Input: part model. Units: mm. Frame: model coordinates. A direction names the side the tool comes from. Coordinates: 2 decimals unless noted, no trailing zeros. Loops run counter-clockwise (first coordinate to the right, second up) from the corner with the lowest first, then second, coordinate; pieces in that order, holes last.
Item 1: Reachability of faces 5 (the flat face through (-9.55, 41, 12)), 6 (the cylindrical face through (-17.435, 32.128, 3.838)), 7 (the flat face through (-6, 26, 10)), 8 (the flat face through (-3.032, 41, 7)) from +Z, -Z, +X, -X, +Y, -Y: full face, straight path, thin tool, end or side. Return the list, or none.
Item 2: Section D-D on z = 1.25. Return loops of the section in (x, y), and give its area (3 significant figures).
Item 3: Section B-B on y = 41. Return loops of the section in (x, z).
Item 4: Section A-A on z = 9.85. Return loops of the section in (x, y), and give its area (3 significant figures).
Item 5: Pull-direction query (Z, two-part tool) for faces 1 (the cylindrical face through (-6.337, 41.26, 11.833)), 2 (the flat face through (0.45, -4, 2)), 3 (the flat face through (-6, 41, 15)), 4 (the flat face through (-20, 16, 0)); classes: released by +Z, released by -Z, zero draft, split by the parting line, or undercut.
Item 6: Section C-C on x = -22.5. Return loops of the section in (y, z), and give its area (3 significant figures).
Item 7: Ray query, line 1 along Y through (x, z) = (-4, 6.75); line 2 along Y through (x, z) = (-3.5, 14.5); line 3 along Z through (x, y) = (-16, -2.5). Return the intervals inside material, ascending.
Item 8: Contact query for flat-ended pins moving along their axis: P1, Ø1.3, axis at y = 29, z = 10.5, coming from the +X side; P2, Ø7, axis at x = -5, z = 9, coming from the -Y side; P3, Ø18, axis at x = -22.05, y = 41, coming from the +Z side. Output: stop coordinate, or through.
```python
from build123d import *

# Parameters (mm, degrees)
F0_R       = 3.5
F0_R_2     = 10
F0_R_3     = 2
F1_DEPTH   = 4.7
F2_SIZE2   = 1.6781992624
F2_SIZE    = 2
F2_2_SIZE2 = 1.6781992624
F2_2_SIZE  = 2
F2_3_SIZE2 = 1.6781992624
F2_3_SIZE  = 2
F3_DEPTH   = 15
F0_R_4     = 4.75
F4_DEPTH   = 3
F5_R       = 2
F6_DEPTH   = 8


# Not quite as in the source:
# - a feature names something its author has since deleted; it is built from what else it names


with BuildPart() as f1:
    # F0 (on Top) → F1 (new body)
    with BuildSketch(Plane.XY):
        Polygon((-39.2612926662, 18.4351751247), (-14.0709569678, -26), (0.450202167, -26), (0.450202167, 18.6235290021), (-3.0323355459, 26), (-9.549797833, 26), (-9.549797833, 56), (-39.2612926662, 56), align=None)
        with Locations((-7.549797833, -21)):
            Circle(F0_R, mode=Mode.SUBTRACT)
        with Locations((-28.549797833, 21)):
            Circle(F0_R, mode=Mode.SUBTRACT)
        with Locations((-22.049797833, 41)):
            Circle(F0_R_2, mode=Mode.SUBTRACT)
        with Locations((-9.549797833, 21)):
            Circle(F0_R, mode=Mode.SUBTRACT)
        with BuildLine():
            Line((-9.549797833, 26), (-3.0323355459, 26))
            Line((-3.0323355459, 26), (-3.0323355459, 30.2973261729))
            ThreePointArc((-3.0323355459, 30.2973261729), (-5.399797833, 33.5), (-3.0323355459, 36.7026738271))
            Line((-3.0323355459, 36.7026738271), (-3.0323355459, 45.2973261729))
            ThreePointArc((-3.0323355459, 45.2973261729), (-5.399797833, 48.5), (-3.0323355459, 51.7026738271))
            Line((-3.0323355459, 51.7026738271), (-3.0323355459, 56))
            Line((-3.0323355459, 56), (-9.549797833, 56))
            Line((-9.549797833, 56), (-9.549797833, 26))
        make_face()
        with Locations((-28.549797833, 21)):
            Circle(F0_R)
        with Locations((-28.549797833, 21)):
            Circle(F0_R_3, mode=Mode.SUBTRACT)
        with Locations((-9.549797833, 21)):
            Circle(F0_R)
        with Locations((-9.549797833, 21)):
            Circle(F0_R_3, mode=Mode.SUBTRACT)
        with Locations((-7.549797833, -21)):
            Circle(F0_R)
        with Locations((-7.549797833, -21)):
            Circle(F0_R_3, mode=Mode.SUBTRACT)
    extrude(amount=F1_DEPTH)

    # F2
    f2_edges = [f1.edges().sort_by_distance(p)[0] for p in [
        (-30.549798, 21, 4.7),
    ]]
    f2_side = f1.faces().sort_by_distance((-30.549798, 21, 2.35))[0]
    chamfer(f2_edges, length=F2_SIZE, length2=F2_SIZE2, reference=f2_side)

    # F2#2
    f2_2_edges = [f1.edges().sort_by_distance(p)[0] for p in [
        (-11.549798, 21, 4.7),
    ]]
    f2_2_side = f1.faces().sort_by_distance((-11.549798, 21, 2.35))[0]
    chamfer(f2_2_edges, length=F2_2_SIZE, length2=F2_2_SIZE2, reference=f2_2_side)

    # F2#3
    f2_3_edges = [f1.edges().sort_by_distance(p)[0] for p in [
        (-9.549798, -21, 4.7),
    ]]
    f2_3_side = f1.faces().sort_by_distance((-9.549798, -21, 2.35))[0]
    chamfer(f2_3_edges, length=F2_3_SIZE, length2=F2_3_SIZE2, reference=f2_3_side)

    # F0 (on Top) → F3 (join)
    with BuildSketch(Plane.XY):
        with BuildLine():
            Line((-9.549797833, 26), (-3.0323355459, 26))
            Line((-3.0323355459, 26), (-3.0323355459, 30.2973261729))
            ThreePointArc((-3.0323355459, 30.2973261729), (-5.399797833, 33.5), (-3.0323355459, 36.7026738271))
            Line((-3.0323355459, 36.7026738271), (-3.0323355459, 45.2973261729))
            ThreePointArc((-3.0323355459, 45.2973261729), (-5.399797833, 48.5), (-3.0323355459, 51.7026738271))
            Line((-3.0323355459, 51.7026738271), (-3.0323355459, 56))
            Line((-3.0323355459, 56), (-9.549797833, 56))
            Line((-9.549797833, 56), (-9.549797833, 26))
        make_face()
    extrude(amount=F3_DEPTH)

    # F0 (on Top) → F4 (join)
    with BuildSketch(Plane.XY):
        with Locations((-22.049797833, 41)):
            Circle(F0_R_2)
        with Locations((-22.049797833, 41)):
            Circle(F0_R_4, mode=Mode.SUBTRACT)
    extrude(amount=F4_DEPTH)

    # F5 (on face) → F6 (cut)
    with BuildSketch(Plane(origin=(-9.549797833, 0, 0), x_dir=(0, -1, 0), z_dir=(-1, 0, 0))):
        with Locations((-41, 9.85)):
            Circle(F5_R)
    extrude(amount=-F6_DEPTH, mode=Mode.SUBTRACT)


solid = f1.part
```
Results found:
1. face 5: +Z, -X, +Y, -Y
1. face 6: +Z
1. face 7: +Z, +X, -X, -Y
1. face 8: +Z, -Z, +X, +Y
2. outline: (-39.26, 18.44) - (-14.07, -26) - (0.45, -26) - (0.45, 18.62) - (-3.03, 26) - (-3.03, 30.3) arc R3.35 cw to (-3.03, 36.7) - (-3.03, 45.3) arc R3.35 cw to (-3.03, 51.7) - (-3.03, 56) - (-39.26, 56) - close; hole circle Ø4 at (-28.55, 21); hole circle Ø9.5 at (-22.05, 41); hole circle Ø4 at (-9.55, 21); hole circle Ø4 at (-7.55, -21)
2. area: 2,450 mm2
3. outline: (-39.26, 0) - (-26.8, 0) - (-26.8, 3) - (-32.05, 3) - (-32.05, 4.7) - (-39.26, 4.7) - close; (-17.3, 0) - (-3.03, 0) - (-3.03, 7.85) - (-9.55, 7.85) - (-9.55, 4.7) - (-12.05, 4.7) - (-12.05, 3) - (-17.3, 3) - close; (-9.55, 11.85) - (-3.03, 11.85) - (-3.03, 15) - (-9.55, 15) - close
4. outline: (-9.55, 26) - (-3.03, 26) - (-3.03, 30.3) arc R3.35 cw to (-3.03, 36.7) - (-3.03, 39) - (-9.55, 39) - close; (-9.55, 43) - (-3.03, 43) - (-3.03, 45.3) arc R3.35 cw to (-3.03, 51.7) - (-3.03, 56) - (-9.55, 56) - close
4. area: 147 mm2
5. face 1: undercut
5. face 2: zero draft
5. face 3: released by +Z
5. face 4: released by -Z
6. outline: (-11.13, 0) - (36.27, 0) - (36.27, 3) - (31.01, 3) - (31.01, 4.7) - (-11.13, 4.7) - close; (45.73, 0) - (56, 0) - (56, 4.7) - (50.99, 4.7) - (50.99, 3) - (45.73, 3) - close
6. area: 253 mm2
7. line 1: y = 26 to 30.78, 36.22 to 45.78, 51.22 to 56
7. line 2: y = 26 to 30.48, 36.52 to 45.48, 51.52 to 56
7. line 3: z = 0 to 4.7
8. P1: stops at x = -3.03
8. P2: stops at y = 26
8. P3: stops at z = 3
